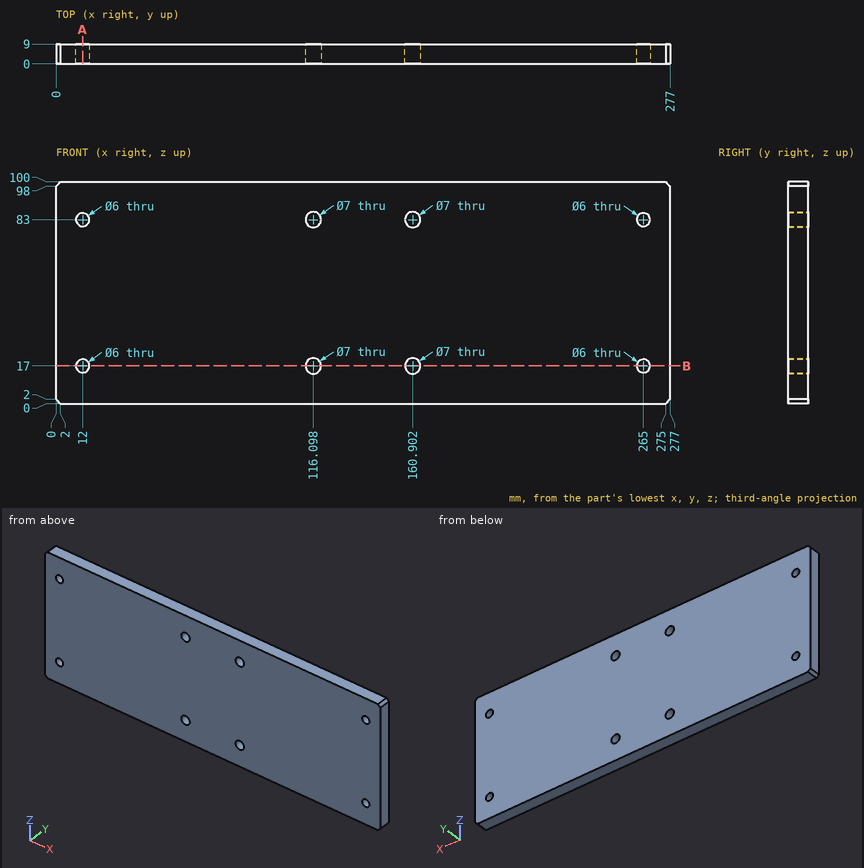
Part print with two shaded views. Sizes in mm from the minimum x, y, z corner. Round coordinates to 2 decimals unless told otherwise and drop trailing zeros. Order: outer loops, then holes, each group sorted by start corner. A loop starts at its lowest first (then second) coordinate and runs counter-clockwise, first axis right, second up. Notation, with made-up numbers: (13.25, 73.25) -> (35.25, 73.25) arc R33 ccw to (35.25, 105.25) -> close; hole circle Ø2 at (6.5, 4.5). An arc over 180 degrees is marked (long way). Use one line per item in the form item = value.
Item 1: Flat gauge pin, fed straight in: pin 1 Ø4 at (x, z) = (160.9, 83) entering from -Y. Where does the tip first touch, or does it go through?
Returned:
pin_1 = through
Item 2: Cut at A-A, the plane x = 12. Write the cut outline in (y, z).
Returned:
outline = (0, 0) -> (9, 0) -> (9, 14) -> (0, 14) -> close; (0, 20) -> (9, 20) -> (9, 80) -> (0, 80) -> close; (0, 86) -> (9, 86) -> (9, 100) -> (0, 100) -> close
Item 3: Drill centre lines: line 1 (Z direction, x = 265, y = 2.5); line 2 (X direction, y = 6.5, z = 19.5). Where is each one in solid material? Low to high.
Returned:
line_1 = 0 to 14, 20 to 80, 86 to 100
line_2 = 0 to 10.34, 13.66 to 113.65, 118.55 to 158.45, 163.35 to 263.34, 266.66 to 277
Item 4: Cut at B-B, the plane z = 17. Write the cut outline in (x, y), and give its area (3 significant figures).
Returned:
outline = (0, 0) -> (9, 0) -> (9, 9) -> (0, 9) -> close; (15, 0) -> (112.6, 0) -> (112.6, 9) -> (15, 9) -> close; (119.6, 0) -> (157.4, 0) -> (157.4, 9) -> (119.6, 9) -> close; (164.4, 0) -> (262, 0) -> (262, 9) -> (164.4, 9) -> close; (268, 0) -> (277, 0) -> (277, 9) -> (268, 9) -> close
area = 2,260 mm^2
